Read the model definition and answer for the solid it produces. Units are mm, in the model's axes. Coordinates: 2 decimals unless noted, no trailing zeros. Loops run counter-clockwise (first coordinate to the right, second up) from the corner with the lowest first, then second, coordinate; pieces in that order, holes last. Notation, with made-up numbers: (28, 80) - (59, 80) arc R13 ccw to (59, 94) - close; hole circle Ø5 at (-32.75, 16.5). An arc over 180 degrees is marked (long way). Use one line per item in the form item = value. Start each with the question number.
1) A cutting plane is placed at B-B (x = -12). Give the vertices of the cut face in (y, z), and give its area (3 significant figures).
2) A cutting plane is placed at A-A (y = 13). Give the vertices of the cut face in (x, z).
3) The mould has two halves that part along Z. Classify faces 1 (the face through (-6.74, 2.12, 7.83)), 2 (the face through (6.2, -1.9, 0)): released by +Z, released by -Z, zero draft, split by the parting line, or undercut.
4) Consider line 1 (Y direction, x = 11, z = 19.5); line 2 (X direction, y = 1, z = 71.5); line 3 (Y direction, x = -4, z = 10.5). Determine where each line is inside the solid, lowest interval first.
5) Each of these flat-tipped pins is pushed along its axis until it touches: P1, Ø1.5, axis at x = 1.5, z = 25.5, coming from the -Y side; P2, Ø12, axis at x = -15, z = 13, coming from the +Y side; P3, Ø4, axis at y = -11.5, z = 27.5, coming from the +X side; P4, Ø10, axis at x = -12, y = -0.5, coming from the -Z side. Where does it stop, or does it pass through?
from build123d import *

# Parameters (mm, degrees)
F3_DEPTH = 1.5
F5_DEPTH = 1.5


with BuildPart() as f1:
    # F0 (on Front) → F1 (revolve)
    with BuildSketch(Plane.XZ):
        with BuildLine():
            Line((0, 7.858783), (0, 74.902989))
            ThreePointArc((0, 74.902989), (-5.978692, 63.096734), (-9.692378, 50.394728))
            ThreePointArc((-9.692378, 50.394728), (-9.455717, 50.045984), (-9.803969, 49.808601))
            ThreePointArc((-9.803969, 49.808601), (-10.770827, 42.605238), (-11.005552, 35.341068))
            ThreePointArc((-11.005552, 35.341068), (-10.745659, 35.091827), (-10.994439, 34.831492))
            ThreePointArc((-10.994439, 34.831492), (-9.647742, 22.685898), (-6.263778, 10.943758))
            Line((-6.263778, 10.943758), (-9.081526, 0))
            Line((-9.081526, 0), (-6.263778, 0))
            Line((-6.263778, 0), (-4.387327, 7.858783))
            Line((-4.387327, 7.858783), (0, 7.858783))
        make_face()
    revolve(axis=Axis((0, 0, 37.451494), (0, 0, -1)))

    # F2 (on Front) → F3 (join, symmetric)
    with BuildSketch(Plane.XZ):
        with BuildLine():
            Line((0, 23.151334), (0, 32.29171))
            ThreePointArc((0, 32.29171), (-17.682558, 20.486984), (-23.366563, 0))
            ThreePointArc((-23.366563, 0), (-13.853883, 13.766447), (0, 23.151334))
        make_face()
        with BuildLine():
            ThreePointArc((23.366563, 0), (17.682558, 20.486984), (0, 32.29171))
            Line((0, 32.29171), (0, 23.151334))
            ThreePointArc((0, 23.151334), (13.853883, 13.766447), (23.366563, 0))
        make_face()
    extrude(amount=F3_DEPTH, both=True)

    # F4 (on Right) → F5 (join, symmetric)
    with BuildSketch(Plane.YZ):
        with BuildLine():
            Line((0, 22.467051), (0, 32.705024))
            ThreePointArc((0, 32.705024), (-17.108651, 20.431419), (-22.198293, 0))
            ThreePointArc((-22.198293, 0), (-13.549792, 13.654856), (0, 22.467051))
        make_face()
        with BuildLine():
            ThreePointArc((22.198293, 0), (17.108651, 20.431419), (0, 32.705024))
            Line((0, 32.705024), (0, 22.467051))
            ThreePointArc((0, 22.467051), (13.549792, 13.654856), (22.198293, 0))
        make_face()
    extrude(amount=F5_DEPTH, both=True)


solid = f1.part
Found:
q1.outline = (-1.5, 15.5) - (1.5, 15.5) - (1.5, 26.45) - (-1.5, 26.45) - close
q1.area = 32.8 mm^2
q2.outline = (-1.5, 14.2) - (1.5, 14.2) - (1.5, 25.3) - (-1.5, 25.3) - close
q3.face_1 = undercut
q3.face_2 = released by -Z
q4.line_1 = -1.5 to 1.5
q4.line_2 = -1.74 to 1.74
q4.line_3 = -4.97 to 4.97
q5.P1 = -13.56
q5.P2 = 1.5
q5.P3 = 4.35
q5.P4 = 0
